Design review of the part built by this model. Coordinates are the model's own, in mm. Face numbers are marked on the shaded views. A direction names the side the tool comes from. Coordinates: 2 decimals unless noted, no trailing zeros. Loops run counter-clockwise (first coordinate to the right, second up) from the corner with the lowest first, then second, coordinate; pieces in that order, holes last.
Q1. Machinability: for the marked faces 1, 2 and 3, which of the approach directions +Z, -Z, +X, -X, +Y, -Y give a long, thin tool a straight path to every point of the face, cutting with its end or side? Answer none if there is none.
Q2. Draft analysis for pull direction Y (two halves, no side actions). For the marked faces 4, 5 and 6, state which applies: released by +Y, released by -Y, zero draft, split by the parting line, or undercut.
Q3. For P1, Ø3, axis at x = -43.5, z = 17.5, coming from the +Y side; P2, Ø1, axis at x = -43, z = 9, coming from the -Y side; P3, Ø2, axis at y = -33.5, z = 19.5, coming from the +X side, all flat-tipped, find the tip position at first contact; note any pin that passes through.
Q4. Add section D-D on x = -71.5. Give the boundary of the cut face in (y, z), and give its area (3 significant figures).
Q5. Add section B-B on y = -27. Give the boundary of the cut face in (x, z), and give its area (3 significant figures).
Q6. Wall thickness on probe 1 along X at (y, z) = (-27.25, 25); probe 2 along Z at (x, y) = (-56, -31.5); probe 3 along Y at (x, z) = (-11.5, 28.5): over which ranges is each line inside the solid? List them lowest first.
Q7. Add section A-A on x = -61.5. Give the boundary of the cut face in (y, z), and give its area (3 significant figures).
Q8. Add section C-C on z = 42. Give the boundary of the cut face in (x, y), and give its area (3 significant figures).
```python
from build123d import *

# Parameters (mm, degrees)
BOSS_EXTRUDE1_START     = 1
SKETCH1_R               = 7
BOSS_EXTRUDE1_DEPTH     = 52
CUT_EXTRUDE1_START      = -18
SKETCH2_R               = 26
CUT_EXTRUDE1_DEPTH      = 6
CUT_EXTRUDE2_DEPTH      = 99.230596048
CUT_EXTRUDE2_DEPTH_BACK = 99.230596048
SKETCH3_R               = 2


with BuildPart() as part:
    # Sketch1 → Boss-Extrude1 (new body)
    with BuildSketch(Plane.XY.offset(BOSS_EXTRUDE1_START)):
        with BuildLine():
            ThreePointArc((-64.866750419, -17), (-83.5, -27), (-64.866750419, -37))
            Line((-64.866750419, -37), (-18.133249581, -37))
            ThreePointArc((-18.133249581, -37), (0.5, -27), (-18.133249581, -17))
            Line((-18.133249581, -17), (-64.866750419, -17))
        make_face()
        with Locations(Location((-71.5, -27, 0), (0, 0, 180))):
            Circle(SKETCH1_R, mode=Mode.SUBTRACT)
        with Locations(Location((-11.5, -27, 0), (0, 0, 180))):
            Circle(SKETCH1_R, mode=Mode.SUBTRACT)
    extrude(amount=BOSS_EXTRUDE1_DEPTH)

    # Sketch2 → Cut-Extrude1 (cut)
    with BuildSketch(Plane.XY.offset(53).offset(CUT_EXTRUDE1_START)):
        with Locations((-71.5, -27)):
            Circle(SKETCH2_R)
    extrude(amount=CUT_EXTRUDE1_DEPTH, mode=Mode.SUBTRACT)

    # Sketch3 → Cut-Extrude2 (cut, two sides: drawn at the far end of the back side and taken through both)
    with BuildSketch(Plane.XY.offset(35).offset(-CUT_EXTRUDE2_DEPTH_BACK)):
        with Locations((-53.61145618, -27)):
            Circle(SKETCH3_R)
    extrude(amount=CUT_EXTRUDE2_DEPTH + CUT_EXTRUDE2_DEPTH_BACK, mode=Mode.SUBTRACT)


solid = part.part
```
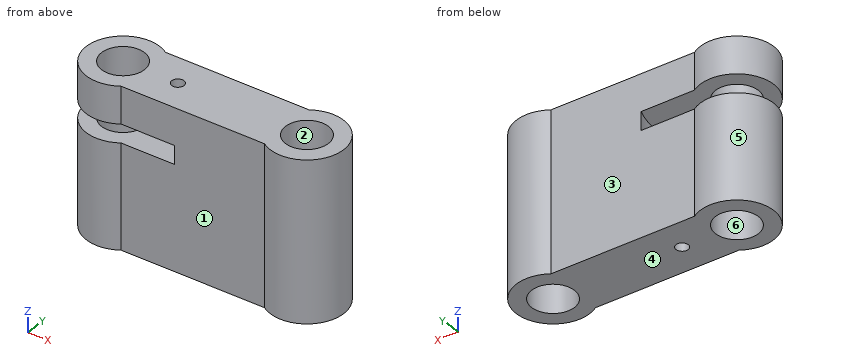
Entries:
1. face 1: +Z, -Z, -Y
1. face 2: +Z, -Z
1. face 3: +Z, -Z, +Y
2. face 4: zero draft
2. face 5: split by the parting line
2. face 6: undercut
3. P1: stops at y = -17
3. P2: stops at y = -37
3. P3: stops at x = -0.83
4. outline: (-39, 1) - (-34, 1) - (-34, 35) - (-39, 35) - close; (-39, 41) - (-34, 41) - (-34, 53) - (-39, 53) - close; (-20, 1) - (-15, 1) - (-15, 35) - (-20, 35) - close; (-20, 41) - (-15, 41) - (-15, 53) - (-20, 53) - close
4. area: 460 mm2
5. outline: (-83.5, 1) - (-78.5, 1) - (-78.5, 35) - (-83.5, 35) - close; (-83.5, 41) - (-78.5, 41) - (-78.5, 53) - (-83.5, 53) - close; (-64.5, 1) - (-55.61, 1) - (-55.61, 35) - (-64.5, 35) - close; (-64.5, 41) - (-55.61, 41) - (-55.61, 53) - (-64.5, 53) - close; (-51.61, 1) - (-18.5, 1) - (-18.5, 53) - (-51.61, 53) - (-51.61, 41) - (-45.5, 41) - (-45.5, 35) - (-51.61, 35) - close; (-4.5, 1) - (0.5, 1) - (0.5, 53) - (-4.5, 53) - close
5. area: 2,580 mm2
6. probe 1: x = -83.5 to -78.5, -64.5 to -55.6, -51.63 to -18.5, -4.5 to 0.5
6. probe 2: z = 1 to 35, 41 to 53
6. probe 3: y = -39 to -34, -20 to -15
7. outline: (-37, 1) - (-17, 1) - (-17, 35) - (-37, 35) - close; (-37, 41) - (-17, 41) - (-17, 53) - (-37, 53) - close
7. area: 920 mm2
8. outline: (-64.87, -37) - (-18.13, -37) arc R12 ccw (long way) to (-18.13, -17) - (-64.87, -17) arc R12 ccw (long way) to start; hole circle Ø14 at (-71.5, -27); hole circle Ø4 at (-53.61, -27); hole circle Ø14 at (-11.5, -27)
8. area: 1,370 mm2
